Geometry check sheet. Reference: the model listing, model coordinates, mm. A direction names the side the tool comes from. Give positions to 0.01 mm unless a question says otherwise; leave off trailing zeros. Order: outer loops, then holes, each group sorted by start corner. A loop starts at its lowest first (then second) coordinate and runs counter-clockwise, first axis right, second up. Notation, with made-up numbers: M 41.25,-28.5 L 55.25,-28.5 A18 cw 55.25,1.5 Z; hole C 5.5,49 d5. An arc over 180 degrees is marked long. Use CSV: the item, a comma, the result in double quotes. Start each with the question number.
from build123d import *

# Parameters (mm, degrees)
F0_W     = 50.8
F0_H     = 50.8
F1_DEPTH = 50.8
F2_R     = 12.7
F3_DEPTH = 25.4
F4_R     = 12.7
F5_DEPTH = 99.06
F7_DEPTH = 60.452
F9_DEPTH = 52.7812


with BuildPart() as f1:
    # F0 (on Top) → F1 (new body)
    with BuildSketch(Plane.XY):
        Rectangle(F0_W, F0_H)
    extrude(amount=F1_DEPTH)

    # F2 (on face) → F3 (join)
    with BuildSketch(Plane.XY.offset(50.8)):
        Circle(F2_R)
    extrude(amount=F3_DEPTH)

    # F4 (on face) → F5 (cut)
    with BuildSketch(Plane.YZ.offset(25.4)):
        with Locations((0, 25.4)):
            Circle(F4_R)
    extrude(amount=-F5_DEPTH, mode=Mode.SUBTRACT)

    # F6 (on face) → F7 (cut)
    with BuildSketch(Plane.YZ.offset(25.4)):
        Polygon((25.4, 9.5578852713), (15.8421147287, 9.5578852713), (25.4, 0), align=None)
    extrude(amount=-F7_DEPTH, mode=Mode.SUBTRACT)

    # F8 (on face) → F9 (cut)
    with BuildSketch(Plane.YZ.offset(25.4)):
        with BuildLine():
            Line((-25.4, 50.8), (-25.4, 45.5264649071))
            add(Edge.make_bspline(
                [(-25.4, 45.5264649071), (-25.015397773, 46.373642787), (-23.3269839792, 48.9886268104), (-20.1866213816, 50.2950406875), (-17.4815941819, 50.8)],
                knots=[0.4167679889, 0.4167679889, 0.4167679889, 0.4167679889, 0.4909297507, 0.6737476918, 0.6737476918, 0.6737476918, 0.6737476918], degree=3))
            Line((-17.4815941819, 50.8), (-25.4, 50.8))
        make_face()
    extrude(amount=-F9_DEPTH, mode=Mode.SUBTRACT)


solid = f1.part
(1) Sectioned sample at C-C on z = 56.5. Record the cut outline in (x, y).
(2) Sectioned sample at B-B on y = 0. Record the cut outline in (x, z).
(3) Thickness scan on line 1 (Z direction, x = -3, y = 0); line 2 (Z direction, x = 15.5, y = 0); line 3 (Y direction, x = -18, z = 20). Record the ranges inside material, lowest first.
(4) Sectioned sample at A-A on z = 25.4. Record the cut outline in (x, y).
(5) Go/stop test with flat-tipped pins: P1, Ø1, axis at x = -16, z = 8, coming from the +Y side; P2, Ø12, axis at y = -12, z = 68.5, coming from the +X side; P3, Ø12, axis at x = 17.5, z = 62.5, coming from the -Y side; P4, Ø5, axis at x = -9, y = 22, coming from the -Z side. Record where each tip stops, or that it passes through.
(6) Access from +Z, -Z, +X, -X, +Y, -Y to the whole of each face (thin tool, end or side, straight path). Record for faces 1 (the face through (-2.75, -12.4, 63.32)), 2 (the face through (0.356, 6.827, 36.109)), 3 (the face through (0, 21, 9.558)).
(7) Sectioned sample at D-D on y = -11. Record the cut outline in (x, z), then the cut area to 3 significant figures.
Responses:
1,outline,"C 0,0 d25.4"
2,outline,"M -25.4,0 L 25.4,0 L 25.4,12.7 L -25.4,12.7 Z; M -25.4,38.1 L 25.4,38.1 L 25.4,50.8 L 12.7,50.8 L 12.7,76.2 L -12.7,76.2 L -12.7,50.8 L -25.4,50.8 Z"
3,line 1,"0 to 12.7, 38.1 to 76.2"
3,line 2,"0 to 12.7, 38.1 to 50.8"
3,line 3,"-25.4 to -11.49, 11.49 to 25.4"
4,outline,"M -25.4,-25.4 L 25.4,-25.4 L 25.4,-12.7 L -25.4,-12.7 Z; M -25.4,12.7 L 25.4,12.7 L 25.4,25.4 L -25.4,25.4 Z"
5,P1,"y = 17.9"
5,P2,"x = 11.19"
5,P3,"y = -5.39"
5,P4,"z = 0"
6,face 1,"+Z"
6,face 2,"+X, -X"
6,face 3,"+X, -X, +Y"
7,outline,"M -25.4,0 L 25.4,0 L 25.4,19.05 L -25.4,19.05 Z; M -25.4,31.75 L 25.4,31.75 L 25.4,50.8 L 6.35,50.8 L 6.35,76.2 L -6.35,76.2 L -6.35,50.8 L -25.4,50.8 Z"
7,area,"2,260 mm2"
